```python
from build123d import *

# Parameters (mm, degrees)
F0_R     = 9.525
F1_DEPTH = 19.05
F3_D     = 12.7
F3_DEPTH = 101.6
F3_TIP   = 3.8154649308
F5_D     = 12.7
F5_DEPTH = 254
F5_TIP   = 3.8154649308


with BuildPart() as f1:
    # F0 (on Top) → F1 (new body)
    with BuildSketch(Plane.XY):
        Polygon((-63.5, 50.8), (-63.5, 0), (-63.5, -50.8), (0, -50.8), (63.5, -50.8), (63.5, 0), (63.5, 50.8), (0, 50.8), align=None)
        with Locations((-44.2700514078, -31.75)):
            Circle(F0_R, mode=Mode.SUBTRACT)
        with Locations((44.6299485922, -31.75)):
            Circle(F0_R, mode=Mode.SUBTRACT)
        with BuildLine():
            ThreePointArc((-25.2200514078, 12.7), (-21.5003075289, 21.6802561211), (-12.5200514078, 25.4))
            Line((-12.5200514078, 25.4), (12.8799485922, 25.4))
            ThreePointArc((12.8799485922, 25.4), (21.8602047133, 21.6802561211), (25.5799485922, 12.7))
            Line((25.5799485922, 12.7), (25.5799485922, -12.7))
            ThreePointArc((25.5799485922, -12.7), (21.8602047133, -21.6802561211), (12.8799485922, -25.4))
            Line((12.8799485922, -25.4), (-12.5200514078, -25.4))
            ThreePointArc((-12.5200514078, -25.4), (-21.5003075289, -21.6802561211), (-25.2200514078, -12.7))
            Line((-25.2200514078, -12.7), (-25.2200514078, 12.7))
        make_face(mode=Mode.SUBTRACT)
        with Locations((-44.2700514078, 31.75)):
            Circle(F0_R, mode=Mode.SUBTRACT)
        with Locations((44.6299485922, 31.75)):
            Circle(F0_R, mode=Mode.SUBTRACT)
    extrude(amount=F1_DEPTH)

    # F3 (one way)
    with BuildSketch(Plane.XZ):
        with Locations((0, 9.525)):
            Circle(F3_D / 2)
    extrude(amount=-F3_DEPTH, mode=Mode.SUBTRACT)
    with Locations(Plane.XZ):
        with Locations((0, 9.525)):
            with Locations((0, 0, -(F3_DEPTH + F3_TIP / 2))):  # 118° drill point
                Cone(0, F3_D / 2, F3_TIP, mode=Mode.SUBTRACT)

    # F5
    with Locations(Plane(origin=(0, 0, 0), x_dir=(1, 0, 0), z_dir=(0, 1, 0))):
        with Locations((0, -9.525)):
            Hole(F5_D / 2, depth=F5_DEPTH)
            with Locations((0, 0, -(F5_DEPTH + F5_TIP / 2))):  # 118° drill point
                Cone(0, F5_D / 2, F5_TIP, mode=Mode.SUBTRACT)


solid = f1.part
```
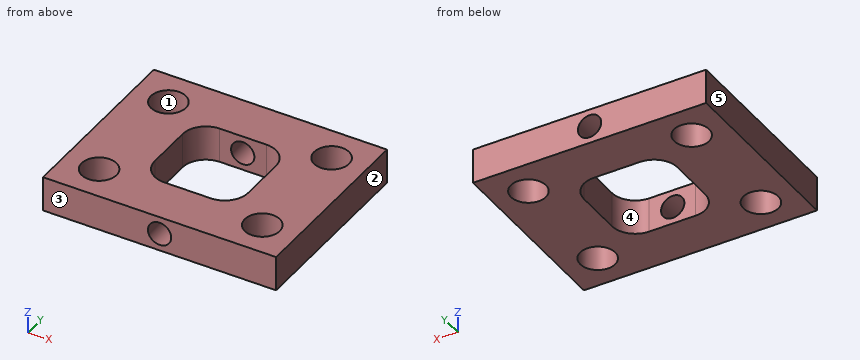
Input: part model. Units: mm. Frame: model coordinates. Face numbers are marked on the shaded views. A direction names the side the tool comes from. Give positions to 0.01 mm unless a question says otherwise; leave off trailing zeros. Loops run counter-clockwise (first coordinate to the right, second up) from the corner with the lowest first, then second, coordinate; pieces in that order, holes last.
1) Section query C-C on z = 7. Return the cut outline in (x, y) (3 decimals).
A:
outline: (-63.5, -50.8) - (-5.826, -50.8) - (-5.826, -25.4) - (-12.52, -25.4) arc R12.7 cw to (-25.22, -12.7) - (-25.22, 12.7) arc R12.7 cw to (-12.52, 25.4) - (-5.826, 25.4) - (-5.826, 50.8) - (-63.5, 50.8) - close; (5.826, -50.8) - (63.5, -50.8) - (63.5, 50.8) - (5.826, 50.8) - (5.826, 25.4) - (12.88, 25.4) arc R12.7 cw to (25.58, 12.7) - (25.58, -12.7) arc R12.7 cw to (12.88, -25.4) - (5.826, -25.4) - close; hole circle Ø19.05 at (-44.27, -31.75); hole circle Ø19.05 at (-44.27, 31.75); hole circle Ø19.05 at (44.63, -31.75); hole circle Ø19.05 at (44.63, 31.75)
2) Contact query for a flat-ended pin moving along its axis: pin 1 (7.5 mm diameter, centred on x = 0, z = 9.525, fed in from +Y). Output: stop coordinate, or through.
A:
pin 1: passes through
3) Section query D-D on y = 7. Return the cut outline in (x, z), and give its area (3 significant figures).
A:
outline: (-63.5, 0) - (-25.22, 0) - (-25.22, 19.05) - (-63.5, 19.05) - close; (25.58, 0) - (63.5, 0) - (63.5, 19.05) - (25.58, 19.05) - close
area: 1,450 mm2
4) Section query A-A on x = 0. Return the cut outline in (y, z) (3 decimals).
A:
outline: (-50.8, 0) - (-25.4, 0) - (-25.4, 3.175) - (-50.8, 3.175) - close; (-50.8, 15.875) - (-25.4, 15.875) - (-25.4, 19.05) - (-50.8, 19.05) - close; (25.4, 0) - (50.8, 0) - (50.8, 3.175) - (25.4, 3.175) - close; (25.4, 15.875) - (50.8, 15.875) - (50.8, 19.05) - (25.4, 19.05) - close
5) Section query B-B on y = -37.5. Return the cut outline in (x, z) (3 decimals), and give its area (3 significant figures).
A:
outline: (-63.5, 0) - (-51.864, 0) - (-51.864, 19.05) - (-63.5, 19.05) - close; (-36.676, 0) - (37.036, 0) - (37.036, 19.05) - (-36.676, 19.05) - close; (52.224, 0) - (63.5, 0) - (63.5, 19.05) - (52.224, 19.05) - close; hole circle Ø12.7 at (0, 9.525)
area: 1,710 mm2
6) Reachability of the marked faces 4 and 5 from +Z, -Z, +X, -X, +Y, -Y: full face, straight path, thin tool, end or side. Return the list, or none.
A:
face 4: +Z, -Z
face 5: +Z, -Z, -X, +Y, -Y
7) Mould query, pull axis X, two halves, no side actions, for the marked faces 1, 2 and 3. Classes: released by +X, released by -X, zero draft, split by the parting line, or undercut.
A:
face 1: undercut
face 2: released by +X
face 3: zero draft
8) Line query: L1, parallel to X at y = 39.5, z = 7.25; L2, parallel to X at y = -32, z = 7; L3, parallel to Z at x = 0, y = -44 (3 decimals). Output: solid intervals per line, ascending.
A:
L1: x = -63.5 to -49.81, -38.73 to -5.93, 5.93 to 39.09, 50.17 to 63.5
L2: x = -63.5 to -53.79, -34.75 to -5.83, 5.83 to 35.11, 54.15 to 63.5
L3: z = 0 to 3.175, 15.875 to 19.05
